```python
from build123d import *

# Parameters (mm, degrees)
F0_R     = 41.5
F0_R_2   = 36.5
F1_DEPTH = 1.6
F2_R     = 36.5
F2_R_2   = 35
F3_DEPTH = 0.95


with BuildPart() as f1:
    # F0 (on Front) → F1 (new body, symmetric)
    with BuildSketch(Plane.XZ):
        Circle(F0_R)
        Circle(F0_R_2, mode=Mode.SUBTRACT)
    extrude(amount=F1_DEPTH, both=True)

    # F2 (on Front) → F3 (join, symmetric)
    with BuildSketch(Plane.XZ):
        Circle(F2_R)
        Circle(F2_R_2, mode=Mode.SUBTRACT)
    extrude(amount=F3_DEPTH, both=True)


solid = f1.part
```
Input: part model. Units: mm. Frame: model coordinates. A direction names the side the tool comes from. Coordinates: 2 decimals unless noted, no trailing zeros. Loops run counter-clockwise (first coordinate to the right, second up) from the corner with the lowest first, then second, coordinate; pieces in that order, holes last. Notation, with made-up numbers: M -3.75,-25 L 43.25,-25 A9 cw 43.25,-10 Z; hole C 41,30.25 d8. An arc over 180 degrees is marked long. Answer in a Markdown table with one row per item.
1. Material intervals for line 1 (Z direction, x = 0, y = -0.2); line 2 (Z direction, x = 0, y = 1.3); line 3 (X direction, y = 1.1, z = -22.5), sorted ascending.
Response:
| item | result |
|---|---|
| line 1 | z = -41.5 to -35, 35 to 41.5 |
| line 2 | z = -41.5 to -36.5, 36.5 to 41.5 |
| line 3 | x = -34.87 to -28.74, 28.74 to 34.87 |
2. Draft query along Z for faces 1 (the flat face through (0, -1.6, -37)), 2 (the flat face through (19, 0.95, -30)), 3 (the cylindrical face through (-28, 0, -21)), 4 (the cylindrical face through (39.584, -0.022, 12.465)). Return one class per face: pulls with the +Z half, pulls with the -Z half, needs draft (parallel to the pull), parting line crosses it, or undercut.
Response:
| item | result |
|---|---|
| face 1 | needs draft |
| face 2 | undercut |
| face 3 | undercut |
| face 4 | parting line crosses it |
3. Reachability of faces 5 (the cylindrical face through (-7.912, 1.28, -35.632)), 6 (the flat face through (0, 1.6, -37)), 7 (the cylindrical face through (-7.912, -1.27, -35.632)) from +Z, -Z, +X, -X, +Y, -Y: full face, straight path, thin tool, end or side. Return the list, or none.
Response:
| item | result |
|---|---|
| face 5 | +Y |
| face 6 | +Z, -Z, +X, -X, +Y |
| face 7 | -Y |
4. Section B-B, the plane x = 0. Output: boundary loops of the cut face in (y, z), then the cut area to 3 significant figures.
Response:
| item | result |
|---|---|
| outline | M -1.6,-41.5 L 1.6,-41.5 L 1.6,-36.5 L 0.95,-36.5 L 0.95,-35 L -0.95,-35 L -0.95,-36.5 L -1.6,-36.5 Z; M -1.6,36.5 L -0.95,36.5 L -0.95,35 L 0.95,35 L 0.95,36.5 L 1.6,36.5 L 1.6,41.5 L -1.6,41.5 Z |
| area | 37.7 mm2 |
5. Section A-A, the plane z = 0. Output: boundary loops of the cut face in (x, y).
Response:
| item | result |
|---|---|
| outline | M -41.5,-1.6 L -36.5,-1.6 L -36.5,-0.95 L -35,-0.95 L -35,0.95 L -36.5,0.95 L -36.5,1.6 L -41.5,1.6 Z; M 35,-0.95 L 36.5,-0.95 L 36.5,-1.6 L 41.5,-1.6 L 41.5,1.6 L 36.5,1.6 L 36.5,0.95 L 35,0.95 Z |
6. First-contact query: pin 1 (10 mm diameter, centred on x = 8.5, z = -29.5, fed in from -Y). Flat tip, straight axial feed; report the tip coordinate or a pass-through.
Response:
| item | result |
|---|---|
| pin 1 | stops at y = -0.95 |
